Part model, mm, in its own coordinate system. A direction names the side the tool comes from. Give positions to 0.01 mm unless a question says otherwise; leave off trailing zeros. Order: outer loops, then holes, each group sorted by start corner. A loop starts at its lowest first (then second) coordinate and runs counter-clockwise, first axis right, second up. Notation, with made-up numbers: (2, 1.5) -> (44, 1.5) arc R21 cw to (44, 22.5) -> close; hole circle Ø6 at (-29, -14.75). An arc over 180 degrees is marked (long way). Write item = value, one per line. Start each with the question number.
Item 1: Band-saw the part on B-B on y = -3. Write the cut outline in (x, z), plus the area to 3 significant figures.
Item 2: Band-saw the part on C-C on y = -20.5. Write the cut outline in (x, z).
Item 3: Tool access for faces 5 (the face through (-30.364, 8, 1)), 6 (the face through (19.036, -8, 1)), 7 (the face through (-26.35, 4.85, 0.99)): list every direction of +Z, -Z, +X, -X, +Y, -Y with a clear straight run to the whole face (end or side of a thin tool).
Item 4: Drill centre lines: line 1 along X through (y, z) = (-24, 1.8); line 2 along X through (y, z) = (-15.5, 0.3); line 3 along Y through (x, z) = (-25.5, 1.6). Where is each one in solid material? Low to high.
Item 5: Band-saw the part on A-A on z = 1.65. Write the cut outline in (x, y).
Item 6: Pull direction Y, two halves, no side cores. Call faces 1 (the face through (23, -21.538, 1)), 2 (the face through (-4, 10.862, 1)), 3 (the face through (-4, -8, 0)), 4 (the face through (23, 5.862, 1)): +Y half, -Y half, draft (parallel to the pull), parting line (faces both ways), or undercut.
Autodesk Inventor part; units mm, degrees
ref_plane "YZ Plane" through (0, 0, 0) normal (1, 0, 0) x (0, 1, 0)
ref_plane "XZ Plane" through (0, 0, 0) normal (0, 1, 0) x (-1, 0, 0)
ref_plane "XY Plane" through (0, 0, 0) normal (0, 0, 1) x (1, 0, 0)
sketch "Sketch1" plane through (0, 0, 0) normal (0, 0, 1) x (1, 0, 0)
  line L0 (-30.3644, 10.862) -> (24.0356, 10.862)
  line L1 (24.0356, 10.862) -> (24.0356, -26.538)
  line L2 (24.0356, -26.538) -> (-30.3644, -26.538)
  line L3 (-30.3644, -26.538) -> (-30.3644, 10.862)
  point P0 (0, 0)
  dimension "d0" = 54.4
  dimension "d1" = 37.4
extrude "Extrusion1" add sketch "Sketch1" along normal blind 2
sketch "Sketch2" plane through (0, 0, 2) normal (0, 0, 1) x (1, 0, 0)
  line L0 (-30.3644, 10.862) -> (24.0356, 10.862)
  line L1 (-30.3644, 10.862) -> (-30.3644, -26.538)
  line L2 (-30.3644, -26.538) -> (24.0356, -26.538)
  line L3 (24.0356, -26.538) -> (24.0356, 10.862)
  point P0 (0, 0)
  point P1 (-27.8644, 8.362)
  point P2 (21.5356, -24.038)
  point P3 (21.5356, 8.362)
  point P4 (-27.8644, -24.038)
  dimension "d4" = 2.5
  dimension "d5" = 2.5
  dimension "d6" = 2.5
  dimension "d7" = 2.5
hole "Hole1" at (-27.8644, 8.362, 2) at (21.5356, -24.038, 2) at (21.5356, 8.362, 2) at (-27.8644, -24.038, 2) direction (0, 0, -1) diameter 2 depth 8 tip angle 118 countersink diameter 4 countersink angle 90
sketch "Sketch3" plane through (0, 0, 2) normal (0, 0, 1) x (1, 0, 0)
  line L0 (-30.3644, -26.538) -> (-30.3644, 10.862)
  line L1 (-30.3644, 5.862) -> (-25.3644, 5.862)
  line L2 (-25.3644, 5.862) -> (-25.3644, -21.538)
  line L3 (-25.3644, -21.538) -> (-30.3644, -21.538)
  line L4 (-30.3644, -21.538) -> (-30.3644, 5.862)
  line L5 (24.0356, 10.862) -> (24.0356, -26.538)
  line L6 (24.0356, 5.862) -> (19.0356, 5.862)
  line L7 (19.0356, 5.862) -> (19.0356, -21.538)
  line L8 (19.0356, -21.538) -> (24.0356, -21.538)
  line L9 (24.0356, -21.538) -> (24.0356, 5.862)
  line L10 (24.0356, 10.862) -> (-30.3644, 10.862)
  line L11 (-30.3644, -26.538) -> (24.0356, -26.538)
  point P0 (0, 0)
  dimension "d15" = 5
  dimension "d16" = 5
  dimension "d17" = 5
  dimension "d18" = 5
extrude "Extrusion2" cut sketch "Sketch3" against normal blind 2 contours L0 L1 L2 L3 | L8 L7 L6 L5
chamfer "Chamfer1" distance 2 angle 45 4 edges at (-25.3644, 5.862, 1) (-25.3644, -21.538, 1) (19.0356, -21.538, 1) (19.0356, 5.862, 1)
properties part number "main body cover"
Values found:
q1.outline = (-25.36, 0) -> (19.04, 0) -> (19.04, 2) -> (-25.36, 2) -> close
q1.area = 88.8 mm^2
q2.outline = (-26.33, 0) -> (20, 0) -> (20, 2) -> (-26.33, 2) -> close
q3.face_5 = +Z, -Z, -X, +Y, -Y
q3.face_6 = +Z, -Z, +X
q3.face_7 = +Z, -Z, -X
q4.line_1 = -30.36 to -29.66, -26.06 to 19.74, 23.34 to 24.04
q4.line_2 = -25.36 to 19.04
q4.line_3 = -26.54 to -19.67, 4 to 10.86
q5.outline = (-30.36, -26.54) -> (24.04, -26.54) -> (24.04, -21.54) -> (21.04, -21.54) -> (19.04, -19.54) -> (19.04, 3.86) -> (21.04, 5.86) -> (24.04, 5.86) -> (24.04, 10.86) -> (-30.36, 10.86) -> (-30.36, 5.86) -> (-27.36, 5.86) -> (-25.36, 3.86) -> (-25.36, -19.54) -> (-27.36, -21.54) -> (-30.36, -21.54) -> close; hole circle Ø3.3 at (-27.86, -24.04); hole circle Ø3.3 at (-27.86, 8.36); hole circle Ø3.3 at (21.54, -24.04); hole circle Ø3.3 at (21.54, 8.36)
q6.face_1 = undercut
q6.face_2 = +Y half
q6.face_3 = draft
q6.face_4 = undercut
